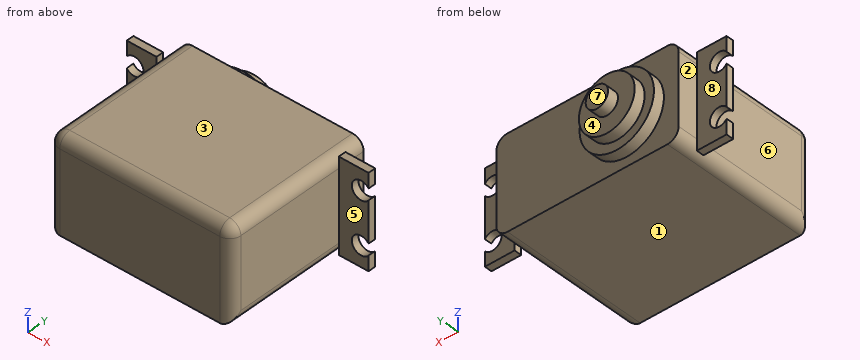
```python
from build123d import *

# Parameters (mm, degrees)
SKETCH1_W           = 49
SKETCH1_H           = 40
BOSS_EXTRUDE1_DEPTH = 25
SKETCH4_R           = 10
BOSS_EXTRUDE2_DEPTH = 3
SKETCH5_R           = 7.5
BOSS_EXTRUDE3_DEPTH = 3
SKETCH6_R           = 3
BOSS_EXTRUDE4_DEPTH = 3
FILLET1_R           = 3
BOSS_EXTRUDE5_DEPTH = 2


with BuildPart() as part:
    # Sketch1 → Boss-Extrude1 (new body)
    with BuildSketch(Plane.XY):
        Rectangle(SKETCH1_W, SKETCH1_H)
    extrude(amount=BOSS_EXTRUDE1_DEPTH)

    # Sketch4 → Boss-Extrude2 (add)
    with BuildSketch(Plane(origin=(0, 20, 0), x_dir=(1, 0, 0), z_dir=(0, 1, 0))):
        with Locations((-10.548196044, -12.468792319)):
            Circle(SKETCH4_R)
    extrude(amount=BOSS_EXTRUDE2_DEPTH)

    # Sketch5 → Boss-Extrude3 (add)
    with BuildSketch(Plane(origin=(0, 23, 0), x_dir=(1, 0, 0), z_dir=(0, 1, 0))):
        with Locations((-10.548196044, -12.468792319)):
            Circle(SKETCH5_R)
    extrude(amount=BOSS_EXTRUDE3_DEPTH)

    # Sketch6 → Boss-Extrude4 (add)
    with BuildSketch(Plane(origin=(0, 26, 0), x_dir=(1, 0, 0), z_dir=(0, 1, 0))):
        with Locations((-10.548196044, -12.468792319)):
            Circle(SKETCH6_R)
    extrude(amount=BOSS_EXTRUDE4_DEPTH)

    # Fillet1
    fillet1_edges = [part.edges().sort_by_distance(p)[0] for p in [
        (24.5, 0, 25),
        (-24.5, 0, 25),
        (24.5, 0, 0),
        (-24.5, 0, 0),
        (0, -20, 25),
        (24.5, -20, 12.5),
        (-24.5, -20, 12.5),
    ]]
    fillet(fillet1_edges, radius=FILLET1_R)

    # Sketch7 → Boss-Extrude5 (add)
    with BuildSketch(Plane(origin=(0, 14.5, 0), x_dir=(1, 0, 0), z_dir=(0, 1, 0))):
        with BuildLine():
            Line((-24.5, 0), (-32.5, 0))
            Line((-32.5, 0), (-32.5, -4))
            ThreePointArc((-32.5, -4), (-28, -5.5), (-32.5, -7))
            Line((-32.5, -7), (-32.5, -18))
            ThreePointArc((-32.5, -18), (-28, -19.5), (-32.5, -21))
            Line((-32.5, -21), (-32.5, -25))
            Line((-32.5, -25), (-24.5, -25))
            Line((-24.5, -25), (-24.5, 0))
        make_face()
        with BuildLine():
            Line((24.5, 0), (24.5, -25))
            Line((24.5, -25), (32.5, -25))
            Line((32.5, -25), (32.5, -21))
            ThreePointArc((32.5, -21), (28, -19.5), (32.5, -18))
            Line((32.5, -18), (32.5, -7))
            ThreePointArc((32.5, -7), (28, -5.5), (32.5, -4))
            Line((32.5, -4), (32.5, 0))
            Line((32.5, 0), (24.5, 0))
        make_face()
    extrude(amount=-BOSS_EXTRUDE5_DEPTH)


solid = part.part
```
Work out the finished part from the listing and answer in its coordinate system (mm). Face numbers are marked on the shaded views. A direction names the side the tool comes from. Give positions to 0.01 mm unless a question says otherwise; leave off trailing zeros. Write each loop counter-clockwise with the first axis right and the second up, starting at its lowest first coordinate (ties: lowest second). Pieces come first, ordered by that corner, then holes.
(1) The part is cut by section B-B on y = -2.5. Write down the section's boundary in (x, z), plus the area to 3 significant figures.
Final values:
outline: (-24.5, 3) arc R3 ccw to (-21.5, 0) - (21.5, 0) arc R3 ccw to (24.5, 3) - (24.5, 22) arc R3 ccw to (21.5, 25) - (-21.5, 25) arc R3 ccw to (-24.5, 22) - close
area: 1,220 mm2
(2) The mould has two halves that part along Z. Classify the marked faces 1, 2 and 3: pulls with the +Z half, pulls with the -Z half, needs draft (parallel to the pull), parting line crosses it, or undercut.
Final values:
face 1: pulls with the -Z half
face 2: needs draft
face 3: pulls with the +Z half
(3) Which of the six approach directions +Z, -Z, +X, -X, +Y, -Y give full straight-line access (tool end or side, diameter ignored) to the marked faces 4, 5, 6, 7 and 8?
Final values:
face 4: +Y
face 5: +Z, -Z, +X, -Y
face 6: +Z, -Z, -X, -Y
face 7: +Z, -Z, +X, -X, +Y
face 8: +Z, -Z, -X, +Y
(4) The part is cut by section D-D on y = 13.5. Write down the section's boundary in (x, z), plus the area to 3 significant figures.
Final values:
outline: (-32.5, 0) - (-24.5, 0) - (-24.5, 3) arc R3 ccw to (-21.5, 0) - (21.5, 0) arc R3 ccw to (24.5, 3) - (24.5, 0) - (32.5, 0) - (32.5, 4) arc R2.5 cw (long way) to (32.5, 7) - (32.5, 18) arc R2.5 cw (long way) to (32.5, 21) - (32.5, 25) - (24.5, 25) - (24.5, 22) arc R3 ccw to (21.5, 25) - (-21.5, 25) arc R3 ccw to (-24.5, 22) - (-24.5, 25) - (-32.5, 25) - (-32.5, 21) arc R2.5 cw (long way) to (-32.5, 18) - (-32.5, 7) arc R2.5 cw (long way) to (-32.5, 4) - close
area: 1,540 mm2
(5) Straight lines are drawn through the part: line 1 (Z direction, x = 30.5, y = 13.7); line 2 (Z direction, x = -30, y = 14); line 3 (X direction, y = 13.45, z = 5.5). For each, find the intervals that lie inside material, in ascending order.
Final values:
line 1: z = 0 to 3, 8 to 17, 22 to 25
line 2: z = 0 to 3.05, 7.95 to 17.05, 21.95 to 25
line 3: x = -28 to 28
(6) Flat-ended cylindrical pins translate along their axes: pin 1 Ø8 at (x, z) = (-30.5, 5.5) entering from -Y; pin 2 Ø4 at (x, z) = (30.5, 19.5) entering from +Y; pin 3 Ø9.5 at (y, z) = (-7, 14.5) entering from +X; pin 4 Ø1 at (x, z) = (-20, 7) entering from +Y. Find the tip coordinate at first contact, or state that the pin passes through.
Final values:
pin 1: stops at y = 12.5
pin 2: passes through
pin 3: stops at x = 24.5
pin 4: stops at y = 20
(7) The part is cut by section C-C on x = -23.5. Write down the section's boundary in (y, z).
Final values:
outline: (-19.24, 0.76) - (20, 0.76) - (20, 24.24) - (-17, 24.24) arc R2.24 ccw to (-19.24, 22) - close
(8) The part is cut by section A-A on x = 30.5. Write down the section's boundary in (y, z), plus the area to 3 significant figures.
Final values:
outline: (12.5, 0) - (14.5, 0) - (14.5, 3) - (12.5, 3) - close; (12.5, 8) - (14.5, 8) - (14.5, 17) - (12.5, 17) - close; (12.5, 22) - (14.5, 22) - (14.5, 25) - (12.5, 25) - close
area: 30.0 mm2
